The listing builds one solid part. Answer for the finished solid, in the listing's coordinates (mm). A direction names the side the tool comes from. Give positions to 0.01 mm unless a question says otherwise; leave off trailing zeros. Order: outer loops, then holes, each group sorted by start corner. A loop starts at its lowest first (then second) coordinate and runs counter-clockwise, first axis right, second up. Notation, with made-up numbers: (-32.75, -15.75) - (8.25, -15.75) arc R24 ccw to (8.25, 12.25) - close; hole circle Ø2 at (46, 54.25). An arc over 180 degrees is marked (long way). Use CSV: the item, a comma, the result in double quotes.
```python
from build123d import *

# Parameters (mm, degrees)
CROQUIS1_R              = 1
SALIENTE_EXTRUIR1_DEPTH = 4
CROQUIS3_R              = 1.25
CORTAR_EXTRUIR1_DEPTH   = 4
CROQUIS4_R              = 1.6
CORTAR_EXTRUIR2_DEPTH   = 4
REDONDEO1_R             = 1.6
CROQUIS5_R              = 1
CORTAR_EXTRUIR3_DEPTH   = 4


with BuildPart() as part:
    # Croquis1 → Saliente-Extruir1 (new body)
    with BuildSketch(Plane.XY):
        with BuildLine():
            Line((-15, -10.656453444), (-15, -40.656453444))
            Line((-15, -40.656453444), (15, -40.656453444))
            Line((15, -40.656453444), (15, -10.656453444))
            ThreePointArc((15, -10.656453444), (0, 18.4), (-15, -10.656453444))
        make_face()
        with Locations((-7.07, 10)):
            Circle(CROQUIS1_R, mode=Mode.SUBTRACT)
        with Locations((7.07, 10)):
            Circle(CROQUIS1_R, mode=Mode.SUBTRACT)
        with Locations((-7.07, 7.9)):
            Circle(CROQUIS1_R, mode=Mode.SUBTRACT)
        with Locations((7.07, 7.9)):
            Circle(CROQUIS1_R, mode=Mode.SUBTRACT)
        with Locations((-7.07, 5.8)):
            Circle(CROQUIS1_R, mode=Mode.SUBTRACT)
        with Locations((7.07, 5.8)):
            Circle(CROQUIS1_R, mode=Mode.SUBTRACT)
        with Locations((-7.07, 3.7)):
            Circle(CROQUIS1_R, mode=Mode.SUBTRACT)
        with Locations((7.07, 3.7)):
            Circle(CROQUIS1_R, mode=Mode.SUBTRACT)
        with Locations((-7.07, 1.6)):
            Circle(CROQUIS1_R, mode=Mode.SUBTRACT)
        with Locations((7.07, 1.6)):
            Circle(CROQUIS1_R, mode=Mode.SUBTRACT)
        with Locations((-7.07, -0.5)):
            Circle(CROQUIS1_R, mode=Mode.SUBTRACT)
        with Locations((7.07, -0.5)):
            Circle(CROQUIS1_R, mode=Mode.SUBTRACT)
        with Locations((-7.07, -2.6)):
            Circle(CROQUIS1_R, mode=Mode.SUBTRACT)
        with Locations((7.07, -2.6)):
            Circle(CROQUIS1_R, mode=Mode.SUBTRACT)
        with Locations((-7.07, -4.7)):
            Circle(CROQUIS1_R, mode=Mode.SUBTRACT)
        with Locations((7.07, -4.7)):
            Circle(CROQUIS1_R, mode=Mode.SUBTRACT)
        with Locations((-7.07, -6.8)):
            Circle(CROQUIS1_R, mode=Mode.SUBTRACT)
        with Locations((7.07, -6.8)):
            Circle(CROQUIS1_R, mode=Mode.SUBTRACT)
        with Locations((-7.07, -8.9)):
            Circle(CROQUIS1_R, mode=Mode.SUBTRACT)
        with Locations((7.07, -8.9)):
            Circle(CROQUIS1_R, mode=Mode.SUBTRACT)
        with Locations((-7.07, -11)):
            Circle(CROQUIS1_R, mode=Mode.SUBTRACT)
        with Locations((7.07, -11)):
            Circle(CROQUIS1_R, mode=Mode.SUBTRACT)
        with Locations((-7.07, -13.1)):
            Circle(CROQUIS1_R, mode=Mode.SUBTRACT)
        with Locations((7.07, -13.1)):
            Circle(CROQUIS1_R, mode=Mode.SUBTRACT)
        with BuildLine():
            Line((3, 0), (3, 10))
            ThreePointArc((3, 10), (0, 13), (-3, 10))
            Line((-3, 10), (-3, 0))
            Line((-3, 0), (-3, -12.5))
            ThreePointArc((-3, -12.5), (0, -15.5), (3, -12.5))
            Line((3, -12.5), (3, 0))
        make_face(mode=Mode.SUBTRACT)
    extrude(amount=SALIENTE_EXTRUIR1_DEPTH)

    # Croquis3 → Cortar-Extruir1 (cut)
    with BuildSketch(Plane.XZ.offset(40.656453444)):
        with Locations(Location((-10, 2, 0), (0, 0, 270))):
            Circle(CROQUIS3_R)
        with Locations(Location((10, 2, 0), (0, 0, 90))):
            Circle(CROQUIS3_R)
    extrude(amount=-CORTAR_EXTRUIR1_DEPTH, mode=Mode.SUBTRACT)

    # Croquis4 → Cortar-Extruir2 (cut)
    with BuildSketch(Plane.XY.offset(4)):
        with Locations((10, -41.656453444)):
            Circle(CROQUIS4_R)
        with Locations((-10, -41.656453444)):
            Circle(CROQUIS4_R)
    extrude(amount=-CORTAR_EXTRUIR2_DEPTH, mode=Mode.SUBTRACT)

    # Redondeo1
    redondeo1_edges = [part.edges().sort_by_distance(p)[0] for p in [
        (15, -10.656453444, 2),
        (-15, -10.656453444, 2),
    ]]
    fillet(redondeo1_edges, radius=REDONDEO1_R)

    # Croquis5 → Cortar-Extruir3 (cut)
    with BuildSketch(Plane.XY.offset(4)):
        with Locations((0, -24.656453444)):
            Circle(CROQUIS5_R)
    extrude(amount=-CORTAR_EXTRUIR3_DEPTH, mode=Mode.SUBTRACT)


solid = part.part
```
Item 1: The part is cut by section D-D (y = -0.5). Give the vertices of the cut face in (x, z).
Taken from the geometry:
outline,"(-18.39, 0) - (-8.07, 0) - (-8.07, 4) - (-18.39, 4) - close; (-6.07, 0) - (-3, 0) - (-3, 4) - (-6.07, 4) - close; (3, 0) - (6.07, 0) - (6.07, 4) - (3, 4) - close; (8.07, 0) - (18.39, 0) - (18.39, 4) - (8.07, 4) - close"
Item 2: The mould has two halves that part along Y. Classify faces 4 (the face through (8.024, -4.4, 1.972)), 5 (the face through (8.024, 8.2, 1.972)), 6 (the face through (-9.98, -40.057, 3.472)), 7 (the face through (11.22, -38.68, 1.73)): +Y half, -Y half, draft (parallel to the pull), parting line (faces both ways), or undercut.
Taken from the geometry:
face 4,"undercut"
face 5,"undercut"
face 6,"-Y half"
face 7,"draft"
Item 3: The part is cut by section C-C (x = -10). Give the vertices of the cut face in (y, z), and give its area (3 significant figures).
Taken from the geometry:
outline,"(-40.06, 0) - (15.45, 0) - (15.45, 4) - (-40.06, 4) - (-40.06, 3.25) - (-36.66, 3.25) - (-36.66, 0.75) - (-40.06, 0.75) - close"
area,"214 mm^2"
Item 4: Find the intervals of material crossed by line 1 along X through (y, z) = (5.5, 3.7); line 2 along X through (y, z) = (-8, 1.55); line 3 along X through (y, z) = (-32.5, 2.9), in increasing order.
Taken from the geometry:
line 1,"-17.56 to -8.02, -6.12 to -3, 3 to 6.12, 8.02 to 17.56"
line 2,"-16.57 to -7.51, -6.63 to -3, 3 to 6.63, 7.51 to 16.57"
line 3,"-15 to 15"
Item 5: The part is cut by section B-B (y = -8.9). Give the vertices of the cut face in (x, z), and give its area (3 significant figures).
Taken from the geometry:
outline,"(-16.1, 0) - (-8.07, 0) - (-8.07, 4) - (-16.1, 4) - close; (-6.07, 0) - (-3, 0) - (-3, 4) - (-6.07, 4) - close; (3, 0) - (6.07, 0) - (6.07, 4) - (3, 4) - close; (8.07, 0) - (16.1, 0) - (16.1, 4) - (8.07, 4) - close"
area,"88.8 mm^2"
Item 6: The part is cut by section A-A (x = -2). Give the vertices of the cut face in (y, z), and give its area (3 significant figures).
Taken from the geometry:
outline,"(-40.66, 0) - (-14.74, 0) - (-14.74, 4) - (-40.66, 4) - close; (12.24, 0) - (18.29, 0) - (18.29, 4) - (12.24, 4) - close"
area,"128 mm^2"
Item 7: Which of the six approach directions +Z, -Z, +X, -X, +Y, -Y give full straight-line access (tool end or side, diameter ignored) to faces 1 (the face through (3, -1, 2)), 2 (the face through (-9.98, -40.057, 0.555)), 3 (the face through (15, -26, 2))?
Taken from the geometry:
face 1,"+Z, -Z"
face 2,"+Z, -Z, -Y"
face 3,"+Z, -Z, +X, -Y"
Item 8: Each of these flat-tipped pins is pushed along its axis until it touches: pin 1 (1.2 mm diameter, centred on y = 1.5, z = 1.5, fed in from +X); pin 2 (5 mm diameter, centred on x = -2.5, y = -0.5, fed in from -Z); pin 3 (1.5 mm diameter, centred on x = -5, z = 2.5, fed in from +Y); pin 4 (1 mm diameter, centred on y = -2.5, z = 2, fed in from +X). Where does it stop, or does it pass through?
Taken from the geometry:
pin 1,"x = 18.38"
pin 2,"z = 0"
pin 3,"y = 17.9"
pin 4,"x = 18.29"
